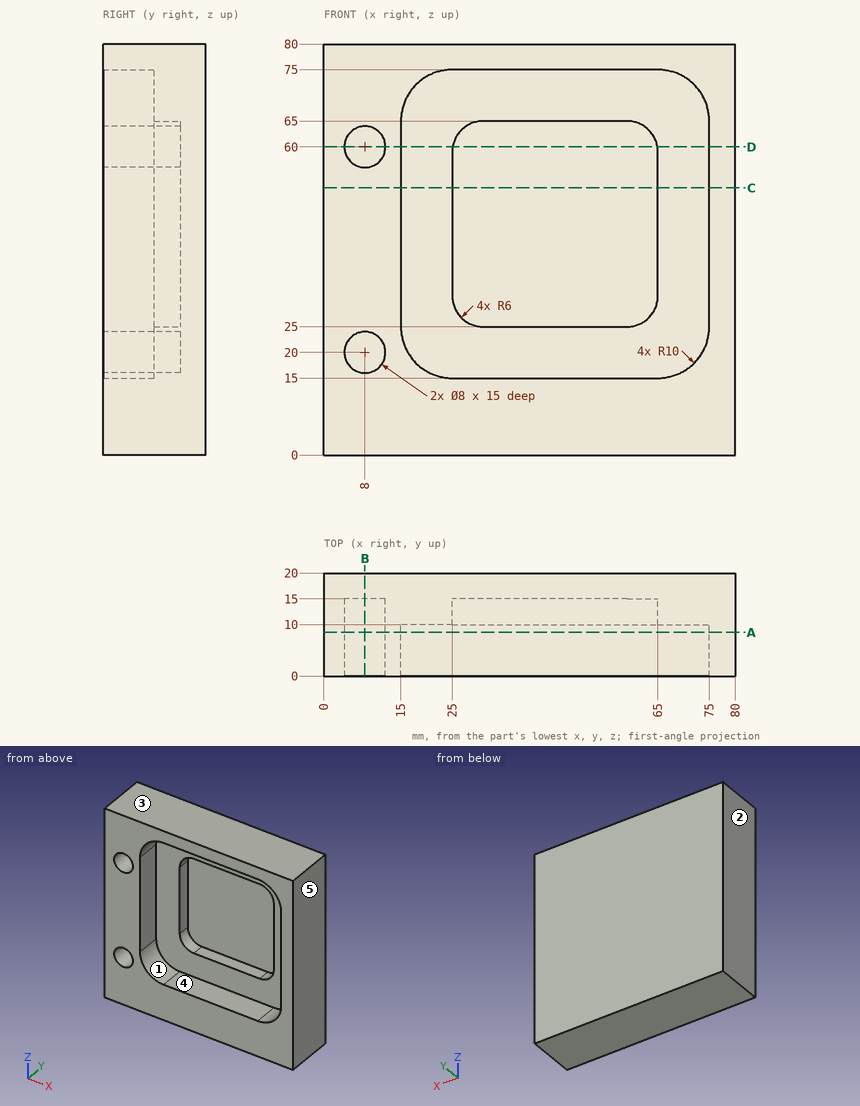
Geometry check sheet. Reference: drawing and pictorial views, mm from the part's lowest x, y, z. A direction names the side the tool comes from. Round coordinates to 2 decimals unless told otherwise and drop trailing zeros. Order: outer loops, then holes, each group sorted by start corner. A loop starts at its lowest first (then second) coordinate and runs counter-clockwise, first axis right, second up. Notation, with made-up numbers: (-5.75, -11) - (10.25, -11) arc R32 cw to (10.25, 22) - close; hole circle Ø11 at (4.25, -9). An arc over 180 degrees is marked (long way). One line per question, with ' | ' between items. Start each with the question number.
(1) Sectioned sample at B-B on x = 8. Record the cut outline in (y, z).
(2) Access from +Z, -Z, +X, -X, +Y, -Y to the whole of each face (thin tool, end or side, straight path). Record for the marked faces 1 and 2.
(3) Thickness scan on L1, parallel to Z at x = 8, y = 5.25; L2, parallel to Z at x = 36, y = 9.5; L3, parallel to Y at x = 56, z = 72. Record the ranges inside material, lowest first. Write a range as [from, to].
(4) Release check for a two-part mould opening along Z. For the marked faces 3, 4 and 5 record: released by +Z, released by -Z, zero draft, split by the parting line, or undercut.
(5) Sectioned sample at C-C on z = 52. Record the cut outline in (x, y).
(6) Sectioned sample at A-A on y = 8.5. Record the cut outline in (x, z), and give its area (3 significant figures).
(7) Depth check by flat-ended pin: pin 1 Ø6 at (x, z) = (55.5, 71.5) entering from -Y; pin 2 Ø12 at (x, z) = (37, 47) entering from -Y. Enter the tip coordinate at first touch or a pass-through.
(8) Sectioned sample at D-D on z = 60. Record the cut outline in (x, y).
Conclusion:
1) outline: (0, 0) - (20, 0) - (20, 80) - (0, 80) - (0, 64) - (15, 64) - (15, 56) - (0, 56) - (0, 24) - (15, 24) - (15, 16) - (0, 16) - close
2) face 1: -Y | face 2: +Z, -Z, -X, +Y, -Y
3) L1: z = [0, 16], [24, 56], [64, 80] | L2: z = [0, 15], [75, 80] | L3: y = [10, 20]
4) face 3: released by +Z | face 4: undercut | face 5: zero draft
5) outline: (0, 0) - (15, 0) - (15, 10) - (25, 10) - (25, 15) - (65, 15) - (65, 10) - (75, 10) - (75, 0) - (80, 0) - (80, 20) - (0, 20) - close
6) outline: (0, 0) - (80, 0) - (80, 80) - (0, 80) - close; hole circle Ø8 at (8, 20); hole circle Ø8 at (8, 60); hole (15, 25) arc R10 ccw to (25, 15) - (65, 15) arc R10 ccw to (75, 25) - (75, 65) arc R10 ccw to (65, 75) - (25, 75) arc R10 ccw to (15, 65) - close | area: 2,790 mm2
7) pin 1: stops at y = 10 | pin 2: stops at y = 15
8) outline: (0, 0) - (4, 0) - (4, 15) - (12, 15) - (12, 0) - (15, 0) - (15, 10) - (25.08, 10) - (25.08, 15) - (64.92, 15) - (64.92, 10) - (75, 10) - (75, 0) - (80, 0) - (80, 20) - (0, 20) - close
